from build123d import *

# Parameters (mm, degrees)
F0_W     = 259.731292
F0_H     = 81.926138
F1_DEPTH = 2.54
F2_DEPTH = 76.2
F4_DEPTH = 3.81
F5_R     = 1.905
F6_DEPTH = 25.4
F7_W     = 2.467993
F7_H     = 69.85
F8_DEPTH = 3.81


with BuildPart() as f1:
    # F0 (on Front) → F1 (new body)
    with BuildSketch(Plane.XZ):
        Rectangle(F0_W, F0_H)
        Polygon((-127, 38.1), (127, 38.1), (127, 0), (127, -38.1), (-127, -38.1), (-127, 0), align=None, mode=Mode.SUBTRACT)
        with BuildLine():
            Line((127, 0), (127, 38.1))
            Line((127, 38.1), (-127, 38.1))
            Line((-127, 38.1), (-127, 0))
            Line((-127, 0), (-121.421141, 0))
            ThreePointArc((-121.421141, 0), (-97.926572, 23.352705), (-74.432003, 0))
            Line((-74.432003, 0), (-63.5, 0))
            Line((-63.5, 0), (-56.090223, 0))
            ThreePointArc((-56.090223, 0), (-32.59841, 23.10803), (-9.106597, 0))
            Line((-9.106597, 0), (0, 0))
            Line((0, 0), (10.213884, 0))
            ThreePointArc((10.213884, 0), (33.708453, 23.352705), (57.203022, 0))
            Line((57.203022, 0), (63.5, 0))
            Line((63.5, 0), (75.297165, 0))
            ThreePointArc((75.297165, 0), (98.740752, 23.597324), (122.286942, 0.10238))
            ThreePointArc((122.286942, 0.10238), (122.286886, 0.05119), (122.286719, 0))
            Line((122.286719, 0), (127, 0))
        make_face()
        with BuildLine():
            Line((127, -38.1), (127, 0))
            Line((127, 0), (122.286719, 0))
            ThreePointArc((122.286719, 0), (98.791942, -23.39262), (75.297165, 0))
            Line((75.297165, 0), (63.5, 0))
            Line((63.5, 0), (57.203022, 0))
            ThreePointArc((57.203022, 0), (57.203345, -0.071147), (57.203453, -0.142295))
            ThreePointArc((57.203453, -0.142295), (33.637305, -23.637187), (10.213884, 0))
            Line((10.213884, 0), (0, 0))
            Line((0, 0), (-9.106597, 0))
            ThreePointArc((-9.106597, 0), (-9.104207, -0.193478), (-9.10341, -0.38697))
            ThreePointArc((-9.10341, -0.38697), (-32.791901, -23.881173), (-56.090223, 0))
            Line((-56.090223, 0), (-63.5, 0))
            Line((-63.5, 0), (-74.432003, 0))
            ThreePointArc((-74.432003, 0), (-74.43168, -0.071147), (-74.431572, -0.142295))
            ThreePointArc((-74.431572, -0.142295), (-97.99772, -23.637187), (-121.421141, 0))
            Line((-121.421141, 0), (-127, 0))
            Line((-127, 0), (-127, -38.1))
            Line((-127, -38.1), (127, -38.1))
        make_face()
    extrude(amount=F1_DEPTH)

    # F0 (on Front) → F2 (join)
    with BuildSketch(Plane.XZ):
        Rectangle(F0_W, F0_H)
        Polygon((-127, 38.1), (127, 38.1), (127, 0), (127, -38.1), (-127, -38.1), (-127, 0), align=None, mode=Mode.SUBTRACT)
    extrude(amount=-F2_DEPTH)

    # F3 (on face) → F4 (join)
    with BuildSketch(Plane.XZ):
        with BuildLine():
            Line((73.582936, 0), (70.973357, 0))
            ThreePointArc((70.973357, 0), (98.843972, -28.284051), (126.990887, -0.274948))
            ThreePointArc((126.990887, -0.274948), (126.99055, -0.137473), (126.989538, 0))
            Line((126.989538, 0), (124.379959, 0))
            ThreePointArc((124.379959, 0), (124.381075, -0.137472), (124.381448, -0.274948))
            ThreePointArc((124.381448, -0.274948), (98.843971, -25.674576), (73.582936, 0))
        make_face()
        with BuildLine():
            ThreePointArc((126.989538, 0), (98.981448, 27.734491), (70.973357, 0))
            Line((70.973357, 0), (73.582936, 0))
            ThreePointArc((73.582936, 0), (98.981448, 25.125052), (124.379959, 0))
            Line((124.379959, 0), (126.989538, 0))
        make_face()
        with BuildLine():
            ThreePointArc((61.736299, 0), (33.727009, 27.91779), (5.717719, 0))
            Line((5.717719, 0), (8.327174, 0))
            ThreePointArc((8.327174, 0), (33.727009, 25.308351), (59.126844, 0))
            Line((59.126844, 0), (61.736299, 0))
        make_face()
        with BuildLine():
            Line((8.327174, 0), (5.717719, 0))
            ThreePointArc((5.717719, 0), (33.681184, -28.101052), (61.736449, -0.091649))
            ThreePointArc((61.736449, -0.091649), (61.736411, -0.045825), (61.736299, 0))
            Line((61.736299, 0), (59.126844, 0))
            ThreePointArc((59.126844, 0), (59.126968, -0.045825), (59.127009, -0.091649))
            ThreePointArc((59.127009, -0.091649), (33.681184, -25.491608), (8.327174, 0))
        make_face()
        with BuildLine():
            ThreePointArc((-58.027052, 0), (-32.627217, 25.308351), (-7.227383, 0))
            Line((-7.227383, 0), (-4.617928, 0))
            ThreePointArc((-4.617928, 0), (-32.627217, 27.91779), (-60.636507, 0))
            Line((-60.636507, 0), (-58.027052, 0))
        make_face()
        with BuildLine():
            ThreePointArc((-7.227383, 0), (-7.227259, -0.045825), (-7.227217, -0.091649))
            ThreePointArc((-7.227217, -0.091649), (-32.673042, -25.491608), (-58.027052, 0))
            Line((-58.027052, 0), (-60.636507, 0))
            ThreePointArc((-60.636507, 0), (-32.673042, -28.101052), (-4.617778, -0.091649))
            ThreePointArc((-4.617778, -0.091649), (-4.617815, -0.045825), (-4.617928, 0))
            Line((-4.617928, 0), (-7.227383, 0))
        make_face()
        with BuildLine():
            ThreePointArc((-70.238811, -0.091649), (-70.238849, -0.045825), (-70.238961, 0))
            Line((-70.238961, 0), (-72.848416, 0))
            ThreePointArc((-72.848416, 0), (-72.848292, -0.045825), (-72.848251, -0.091649))
            ThreePointArc((-72.848251, -0.091649), (-98.294076, -25.491608), (-123.648085, 0))
            Line((-123.648085, 0), (-126.257541, 0))
            ThreePointArc((-126.257541, 0), (-98.294076, -28.101052), (-70.238811, -0.091649))
        make_face()
        with BuildLine():
            Line((-72.848416, 0), (-70.238961, 0))
            ThreePointArc((-70.238961, 0), (-98.248251, 27.91779), (-126.257541, 0))
            Line((-126.257541, 0), (-123.648085, 0))
            ThreePointArc((-123.648085, 0), (-98.248251, 25.308351), (-72.848416, 0))
        make_face()
    extrude(amount=-F4_DEPTH)

    # F5 (on face) → F6 (cut)
    with BuildSketch(Plane.YZ.offset(129.865646)):
        with Locations((24.066546, 0)):
            Circle(F5_R)
    extrude(amount=-F6_DEPTH, mode=Mode.SUBTRACT)

    # F7 (on face) → F8 (join)
    with BuildSketch(Plane(origin=(0, 0, 38.1), x_dir=(1, 0, 0), z_dir=(0, 0, -1))):
        Polygon((-37.20969, -73.142835), (-34.925, -73.142835), (-34.925, -3.292835), (-34.925, -3.207732), (-37.20969, -3.207732), align=None)
        with Locations((36.158997, -38.217835)):
            Rectangle(F7_W, F7_H)
    extrude(amount=F8_DEPTH)


solid = f1.part
Work out the finished part from the listing and answer in its coordinate system (mm). A direction names the side the tool comes from. Give positions to 0.01 mm unless a question says otherwise; leave off trailing zeros. Loops run counter-clockwise (first coordinate to the right, second up) from the corner with the lowest first, then second, coordinate; pieces in that order, holes last. Notation, with made-up numbers: (-16.75, -36.75) -> (15.25, -36.75) arc R7 cw to (15.25, -25.75) -> close; hole circle Ø8 at (-20.5, -38.5). An arc over 180 degrees is marked (long way). Use a Markdown table: item, result. Add a question column.
1) The part is cut by section B-B, the plane x = 29.5. Determine the outline of the cut face in (y, z), plus the area to 3 significant figures.
2) The part is cut by section D-D, the plane z = -10. Count the separate pieces of the cut face and the enclosed holes in it, plus the area to 3 significant figures.
3) Which of the six approach directions +Z, -Z, +X, -X, +Y, -Y give full straight-line access (tool end or side, diameter ignored) to faces 1 (the flat face through (-2, -2.54, 1)), 2 (the flat face through (2, 38, -38.1))?
4) Each of these flat-tipped pins is pushed along its axis until it touches: P1, Ø12, axis at x = -88.5, z = 25, coming from the +Y side; P2, Ø2, axis at x = -33, z = 29, coming from the +Y side. Where does it stop, or does it pass through?
5) For a pull along X with two mould halves and no side action, classify faces 3 (the flat face through (-2, 36, 40.963)), 4 (the flat face through (129.866, 36, -1)), 5 (the flat face through (127, 38, 1)) as +X half, -X half, draft (parallel to the pull), parting line (faces both ways), or undercut.
6) The part is cut by section C-C, the plane z = -35. Determine the outline of the cut face in (x, y).
7) The part is cut by section A-A, the plane y = 15. Determine the outline of the cut face in (x, z) (3 decimals), plus the area to 3 significant figures.
8) Consider line 1 along X through (y, z) = (38, 15); line 2 along Z through (x, y) = (83, 56.5); line 3 along Y through (x, z) = (-51.5, -22). Determine where each line is inside the solid, lowest interval first.
Reported:
| question | item | result |
|---|---|---|
| 1 | outline | (-2.54, -40.96) -> (76.2, -40.96) -> (76.2, -38.1) -> (0, -38.1) -> (0, -27.78) -> (3.81, -27.78) -> (3.81, -25.14) -> (0, -25.14) -> (0, -23.26) -> (-2.54, -23.26) -> close; (-2.54, 22.97) -> (0, 22.97) -> (0, 24.95) -> (3.81, 24.95) -> (3.81, 27.6) -> (0, 27.6) -> (0, 38.1) -> (76.2, 38.1) -> (76.2, 40.96) -> (-2.54, 40.96) -> close |
| 1 | area | 547 mm^2 |
| 2 | separate pieces | 5 |
| 2 | enclosed holes | 0 |
| 2 | area | 749 mm^2 |
| 3 | face 1 | +Z, -Z, +X, -X, -Y |
| 3 | face 2 | +Y |
| 4 | P1 | stops at y = 3.81 |
| 4 | P2 | stops at y = 0 |
| 5 | face 3 | draft |
| 5 | face 4 | +X half |
| 5 | face 5 | undercut |
| 6 | outline | (-129.87, -2.54) -> (129.87, -2.54) -> (129.87, 76.2) -> (127, 76.2) -> (127, 0) -> (-127, 0) -> (-127, 76.2) -> (-129.87, 76.2) -> close |
| 7 | outline | (-129.866, -40.963) -> (129.866, -40.963) -> (129.866, 40.963) -> (-129.866, 40.963) -> close; hole (-127, -38.1) -> (127, -38.1) -> (127, 38.1) -> (37.393, 38.1) -> (37.393, 34.29) -> (34.925, 34.29) -> (34.925, 38.1) -> (-34.925, 38.1) -> (-34.925, 34.29) -> (-37.21, 34.29) -> (-37.21, 38.1) -> (-127, 38.1) -> close |
| 7 | area | 1,940 mm^2 |
| 8 | line 1 | x = -129.87 to -127, 127 to 129.87 |
| 8 | line 2 | z = -40.96 to -38.1, 38.1 to 40.96 |
| 8 | line 3 | y = -2.54 to 0 |
